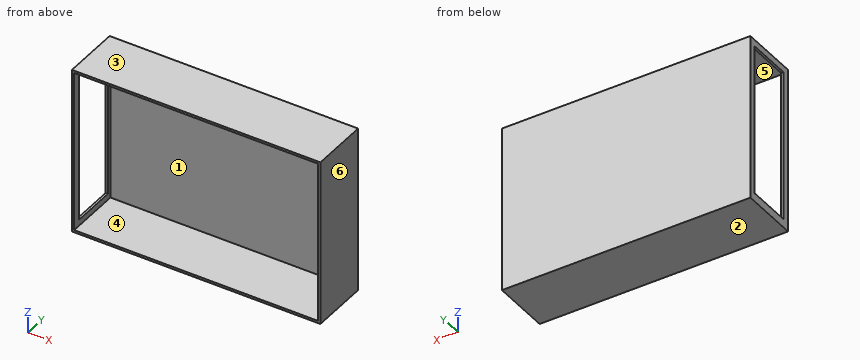
from build123d import *

# Parameters (mm, degrees)
F0_W     = 107.7976
F0_H     = 72.2376
F1_DEPTH = 25.4
F2_T     = -0.9906
F3_W     = 19.471491
F3_H     = 65.671131
F4_DEPTH = 25.4


with BuildPart() as f1:
    # F0 (on Front) → F1 (new body)
    with BuildSketch(Plane.XZ):
        Rectangle(F0_W, F0_H)
    extrude(amount=F1_DEPTH)

    # F2
    f2_openings = [f1.faces().sort_by_distance(p)[0] for p in [
        (0, -25.4, 0),
    ]]
    offset(amount=F2_T, openings=f2_openings)

    # F3 (on face) → F4 (cut)
    with BuildSketch(Plane(origin=(-53.8988, 0, 0), x_dir=(0, -1, 0), z_dir=(-1, 0, 0))):
        with Locations((12.441532, 0.397727)):
            Rectangle(F3_W, F3_H)
    extrude(amount=-F4_DEPTH, mode=Mode.SUBTRACT)


solid = f1.part
The listing builds one solid part. Answer for the finished solid, in the listing's coordinates (mm). Face numbers are marked on the shaded views. A direction names the side the tool comes from. Give positions to 0.01 mm unless a question says otherwise; leave off trailing zeros. Order: outer loops, then holes, each group sorted by start corner. A loop starts at its lowest first (then second) coordinate and runs counter-clockwise, first axis right, second up. Notation, with made-up numbers: (2, 13.25) -> (36, 13.25) arc R26 ccw to (36, 41.25) -> close; hole circle Ø9 at (27, -20.5). An arc over 180 degrees is marked (long way). Put each result on its own line as item: value.
Item 1: A cutting plane is placed at A-A on z = -21. Give the vertices of the cut face in (x, y).
Established:
outline: (-53.9, -25.4) -> (-52.91, -25.4) -> (-52.91, -22.18) -> (-53.9, -22.18) -> close; (-53.9, -2.71) -> (-52.91, -2.71) -> (-52.91, -0.99) -> (52.91, -0.99) -> (52.91, -25.4) -> (53.9, -25.4) -> (53.9, 0) -> (-53.9, 0) -> close
Item 2: For the marked faces 5 and 6, determine the directions among +Z, -Z, +X, -X, +Y, -Y from which every point of the face is accessible in a straight line to the end or side of a thin tool.
Established:
face 5: -Y
face 6: +Z, -Z, +X, +Y, -Y
Item 3: A cutting plane is placed at B-B on y = -11.25. Give the vertices of the cut face in (x, z), plus the area to 3 significant figures.
Established:
outline: (-53.9, -36.12) -> (53.9, -36.12) -> (53.9, 36.12) -> (-53.9, 36.12) -> (-53.9, 33.23) -> (-52.91, 33.23) -> (-52.91, 35.13) -> (52.91, 35.13) -> (52.91, -35.13) -> (-52.91, -35.13) -> (-52.91, -32.44) -> (-53.9, -32.44) -> close
area: 288 mm^2
Item 4: For a pull along Z with two mould halves and no side action, classify the marked faces 1, 2, 3 and 4 as released by +Z, released by -Z, zero draft, split by the parting line, or undercut.
Established:
face 1: undercut
face 2: released by -Z
face 3: released by +Z
face 4: undercut
Item 5: A cutting plane is placed at C-C on x = 13. Give the vertices of the cut face in (y, z).
Established:
outline: (-25.4, -36.12) -> (0, -36.12) -> (0, 36.12) -> (-25.4, 36.12) -> (-25.4, 35.13) -> (-0.99, 35.13) -> (-0.99, -35.13) -> (-25.4, -35.13) -> close
Item 6: Straight lines are drawn through the part: line 1 (Z direction, x = 7, y = -5.25); line 2 (Y direction, x = -31, z = 32); line 3 (X direction, y = -17, z = -17). For each, find the intervals that lie inside material, in ascending order.
Established:
line 1: z = -36.12 to -35.13, 35.13 to 36.12
line 2: y = -0.99 to 0
line 3: x = 52.91 to 53.9
Item 7: Given P1, Ø5, axis at y = -17.5, z = 3, coming from the -X side; P2, Ø12, axis at x = -5, z = 10, coming from the -Y side, each flat-ended and moving along its own axis, determine where each tip first touches the part or whether it passes through.
Established:
P1: stops at x = 52.91
P2: stops at y = -0.99
